Could you check a few things on this model? Use its own coordinates, in mm. Face numbers are marked on the shaded views. A direction names the side the tool comes from. Coordinates: 2 decimals unless noted, no trailing zeros. Loops run counter-clockwise (first coordinate to the right, second up) from the corner with the lowest first, then second, coordinate; pieces in that order, holes last. Notation, with made-up numbers: (12.5, -24.5) - (20.5, -24.5) arc R11 cw to (20.5, -5.5) - close; hole circle Ø4 at (5.25, 33). An arc over 180 degrees is marked (long way). One line per item, written item: value. Start each with the question number.
(1) If we mould it in two halves opening along X, with no side actions, what happens to the marked faces 3 and 4? For each: pulls with the +X half, pulls with the -X half, needs draft (parallel to the pull), parting line crosses it, or undercut.
(2) On a 3-axis mill with a long thin cutter (end or side, diameter ignored), from which of +Z, -Z, +X, -X, +Y, -Y can I reach the whole of each face in a straight line? I mean the marked faces 1 and 2. Say none if no direction works.
(3) I'm going to push a flat-ended pin straight in: P1, Ø6, axis at x = 325.5, z = 209, coming from the +Y side. Where does the tip first touch, or does it pass through?
(4) If we section it at B-B on x = 409.5: Write out the boundary of the cut face in (y, z).
(5) If I drill on line 1 along Y through (x, z) = (266.5, 341.5); line 2 along X through (y, z) = (105, 146) (3 decimals), over which ranges is the centre line in solid material (lowest first)? Write a range as from..to.
(6) If we section it at C-C on z = 202.5: Count the separate pieces of the cut face and the enclosed holes in it, then the cut area to 3 significant figures.
(7) If we section it at A-A on y = 141: Write out the boundary of the cut face in (x, z) (3 decimals).
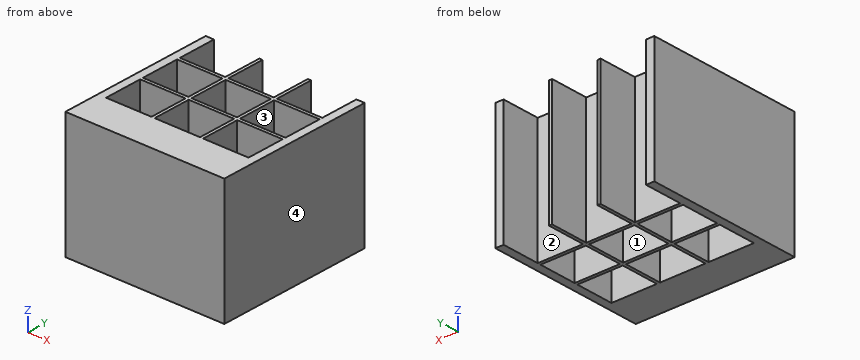
```python
from build123d import *

# Parameters (mm, degrees)
SKETCH1_W           = 137.3
SKETCH1_H           = 9.525
SKETCH1_W_2         = 9.525
SKETCH1_H_2         = 116.877063157
SKETCH1_H_3         = 116.877063158
SKETCH1_W_3         = 480.95
SKETCH1_H_4         = 111.268810527
BOSS_EXTRUDE1_DEPTH = 375


with BuildPart() as part:
    # Sketch1 → Boss-Extrude1 (new body)
    with BuildSketch(Plane.XY):
        Polygon((0, 369.681189473), (0, 0), (25, 0), (25, 116.877063158), (25, 126.402063158), (25, 243.279126316), (25, 252.804126316), (25, 369.681189473), align=None)
        with Locations((93.65, 248.041626316)):
            Rectangle(SKETCH1_W, SKETCH1_H)
        with Locations((167.0625, 248.041626316)):
            Rectangle(SKETCH1_W_2, SKETCH1_H)
        with Locations((167.0625, 311.242657894)):
            Rectangle(SKETCH1_W_2, SKETCH1_H_2)
        with Locations((167.0625, 184.840594737)):
            Rectangle(SKETCH1_W_2, SKETCH1_H_3)
        with Locations((93.65, 121.639563158)):
            Rectangle(SKETCH1_W, SKETCH1_H)
        with Locations((167.0625, 121.639563158)):
            Rectangle(SKETCH1_W_2, SKETCH1_H)
        with Locations((167.0625, 58.438531579)):
            Rectangle(SKETCH1_W_2, SKETCH1_H_3)
        with Locations((240.475, 121.639563158)):
            Rectangle(SKETCH1_W, SKETCH1_H)
        with Locations((240.475, 248.041626316)):
            Rectangle(SKETCH1_W, SKETCH1_H)
        with Locations((313.8875, 311.242657894)):
            Rectangle(SKETCH1_W_2, SKETCH1_H_2)
        with Locations((313.8875, 248.041626316)):
            Rectangle(SKETCH1_W_2, SKETCH1_H)
        with Locations((313.8875, 184.840594737)):
            Rectangle(SKETCH1_W_2, SKETCH1_H_3)
        with Locations((387.3, 248.041626316)):
            Rectangle(SKETCH1_W, SKETCH1_H)
        Polygon((455.95, 0), (480.95, 0), (480.95, 369.681189473), (455.95, 369.681189473), (455.95, 252.804126316), (455.95, 243.279126316), (455.95, 126.402063158), (455.95, 116.877063158), align=None)
        with Locations((387.3, 121.639563158)):
            Rectangle(SKETCH1_W, SKETCH1_H)
        with Locations((313.8875, 121.639563158)):
            Rectangle(SKETCH1_W_2, SKETCH1_H)
        with Locations((313.8875, 58.438531579)):
            Rectangle(SKETCH1_W_2, SKETCH1_H_3)
        with Locations((240.475, -55.634405264)):
            Rectangle(SKETCH1_W_3, SKETCH1_H_4)
    extrude(amount=BOSS_EXTRUDE1_DEPTH)


solid = part.part
```
Values:
1. face 3: undercut
1. face 4: pulls with the +X half
2. face 1: +Z, -Z
2. face 2: +Z, -Z, +Y
3. P1: stops at y = 252.8
4. outline: (-111.27, 0) - (0, 0) - (0, 375) - (-111.27, 375) - close; (116.88, 0) - (126.4, 0) - (126.4, 375) - (116.88, 375) - close; (243.28, 0) - (252.8, 0) - (252.8, 375) - (243.28, 375) - close
5. line 1: y = -111.27..0, 116.88..126.4, 243.28..252.8
5. line 2: x = 0..25, 162.3..171.825, 309.125..318.65, 455.95..480.95
6. separate pieces: 1
6. enclosed holes: 6
6. area: 86,900 mm2
7. outline: (0, 0) - (25, 0) - (25, 375) - (0, 375) - close; (162.3, 0) - (171.825, 0) - (171.825, 375) - (162.3, 375) - close; (309.125, 0) - (318.65, 0) - (318.65, 375) - (309.125, 375) - close; (455.95, 0) - (480.95, 0) - (480.95, 375) - (455.95, 375) - close
